Model file for the job. Use its own axes, mm. Face numbers are marked on the shaded views. A direction names the side the tool comes from. Round coordinates to 2 decimals unless told otherwise and drop trailing zeros. Order: outer loops, then holes, each group sorted by start corner. A loop starts at its lowest first (then second) coordinate and runs counter-clockwise, first axis right, second up. Notation, with made-up numbers: (-4.75, 20) - (54.25, 20) arc R29 cw to (54.25, 56) - close; hole circle Ø9 at (88, 75.5). An arc over 180 degrees is marked (long way). Answer as CSV lines item,"result". Start each with the question number.
1. Band-saw the part on B-B on z = -19.5. List the corners of the cut face in (x, y) (3 decimals).
2. Pull direction X, two halves, no side cores. Call the marked faces 6, 7 and 8: released by +X, released by -X, zero draft, split by the parting line, or undercut.
3. Wall check: line 1 along Z through (x, y) = (26, 30); line 2 along X through (y, z) = (65, -109); line 3 along Y through (x, z) = (8, -41). Give the ranges that are in metal, low to high. Write a range as [from, to].
4. Band-saw the part on A-A on y = 0. List the corners of the cut face in (x, z), then the cut area to 3 significant figures.
5. 3-axis set-ups, long thin cutter, end or side, ignore diameter. For the marked faces 1, 2, 3, 4 and 5: which of +Z, -Z, +X, -X, +Y, -Y reach the whole face in a straight line?
6. Band-saw the part on D-D on y = 53.5. List the corners of the cut face in (x, z).
7. Band-saw the part on C-C on x = 16. State how many separate pieces and enclosed holes the cut face has, then the cut area to 3 significant figures.
8. Pin check, flat tips, straight feed: pin 1 Ø13.5 at (x, y) = (14.5, 131) entering from +Z; pin 2 Ø22.5 at (x, z) = (-6.5, 131.5) entering from -Y; pin 3 Ø1.5 at (x, z) = (26, 98) entering from -Y. Stop position of each tip, or through.
```python
from build123d import *

# Parameters (mm, degrees)
BOSS_EXTRUDE1_DEPTH = 50
SKETCH4_R           = 150
SKETCH4_R_2         = 100
BOSS_EXTRUDE3_DEPTH = 100
CUT_EXTRUDE1_DEPTH  = 120
SKETCH7_R           = 150
SKETCH7_R_2         = 105
BOSS_EXTRUDE6_DEPTH = 4


with BuildPart() as part:
    # Sketch2 → Boss-Extrude1 (new, symmetric)
    with BuildSketch(Plane.YZ):
        with BuildLine():
            Line((-24.368621785, -28.502987077), (-80.352540378, -60.825317547))
            Line((-80.352540378, -60.825317547), (-92.852540378, -39.174682453))
            Line((-92.852540378, -39.174682453), (-36.868621785, -6.852351982))
            ThreePointArc((-36.868621785, -6.852351982), (-37.5, 0), (-36.868621785, 6.852351982))
            Line((-36.868621785, 6.852351982), (-92.852540378, 39.174682453))
            Line((-92.852540378, 39.174682453), (-80.352540378, 60.825317547))
            Line((-80.352540378, 60.825317547), (-24.368621785, 28.502987077))
            ThreePointArc((-24.368621785, 28.502987077), (-18.75, 32.475952642), (-12.5, 35.355339059))
            Line((-12.5, 35.355339059), (-12.5, 100))
            Line((-12.5, 100), (12.5, 100))
            Line((12.5, 100), (12.5, 35.355339059))
            ThreePointArc((12.5, 35.355339059), (18.75, 32.475952642), (24.368621785, 28.502987077))
            Line((24.368621785, 28.502987077), (80.352540378, 60.825317547))
            Line((80.352540378, 60.825317547), (92.852540378, 39.174682453))
            Line((92.852540378, 39.174682453), (36.868621785, 6.852351982))
            ThreePointArc((36.868621785, 6.852351982), (37.5, 0), (36.868621785, -6.852351982))
            Line((36.868621785, -6.852351982), (92.852540378, -39.174682453))
            Line((92.852540378, -39.174682453), (80.352540378, -60.825317547))
            Line((80.352540378, -60.825317547), (24.368621785, -28.502987077))
            ThreePointArc((24.368621785, -28.502987077), (18.75, -32.475952642), (12.5, -35.355339059))
            Line((12.5, -35.355339059), (12.5, -100))
            Line((12.5, -100), (-12.5, -100))
            Line((-12.5, -100), (-12.5, -35.355339059))
            ThreePointArc((-12.5, -35.355339059), (-18.75, -32.475952642), (-24.368621785, -28.502987077))
        make_face()
        Polygon((-14.43375673, -25), (14.43375673, -25), (28.867513459, 0), (14.43375673, 25), (-14.43375673, 25), (-28.867513459, 0), align=None, mode=Mode.SUBTRACT)
    extrude(amount=BOSS_EXTRUDE1_DEPTH, both=True)

    # Sketch4 → Boss-Extrude3 (add)
    with BuildSketch(Plane.YZ.offset(50)):
        with Locations(Location((0, 0, 0), (0, 0, 270))):
            Circle(SKETCH4_R)
        Circle(SKETCH4_R_2, mode=Mode.SUBTRACT)
    extrude(amount=-BOSS_EXTRUDE3_DEPTH)

    # Sketch5 → Cut-Extrude1 (cut)
    with BuildSketch(Plane.YZ.offset(50)):
        with BuildLine():
            ThreePointArc((-70.626450965, 77.697518777), (-40.181760398, 97.007350914), (-5, 104.880884817))
            Line((-5, 104.880884817), (-5, 149.916643506))
            ThreePointArc((-5, 149.916643506), (-57.402514855, 138.581929877), (-102.47154133, 109.542609142))
            Line((-102.47154133, 109.542609142), (-70.626450965, 77.697518777))
        make_face()
        with BuildLine():
            Line((70.626450965, 77.697518777), (102.47154133, 109.542609142))
            ThreePointArc((102.47154133, 109.542609142), (57.402514855, 138.581929877), (5, 149.916643506))
            Line((5, 149.916643506), (5, 104.880884817))
            ThreePointArc((5, 104.880884817), (40.181760398, 97.007350914), (70.626450965, 77.697518777))
        make_face()
        with BuildLine():
            ThreePointArc((149.916643506, 5), (138.581929877, 57.402514855), (109.542609142, 102.47154133))
            Line((109.542609142, 102.47154133), (77.697518777, 70.626450965))
            ThreePointArc((77.697518777, 70.626450965), (97.007350914, 40.181760398), (104.880884817, 5))
            Line((104.880884817, 5), (149.916643506, 5))
        make_face()
        with BuildLine():
            Line((149.916643506, -5), (104.880884817, -5))
            ThreePointArc((104.880884817, -5), (97.007350914, -40.181760398), (77.697518777, -70.626450965))
            Line((77.697518777, -70.626450965), (109.542609142, -102.47154133))
            ThreePointArc((109.542609142, -102.47154133), (138.581929877, -57.402514855), (149.916643506, -5))
        make_face()
        with BuildLine():
            Line((102.47154133, -109.542609142), (70.626450965, -77.697518777))
            ThreePointArc((70.626450965, -77.697518777), (40.181760398, -97.007350914), (5, -104.880884817))
            Line((5, -104.880884817), (5, -149.916643506))
            ThreePointArc((5, -149.916643506), (57.402514855, -138.581929877), (102.47154133, -109.542609142))
        make_face()
        with BuildLine():
            Line((-5, -149.916643506), (-5, -104.880884817))
            ThreePointArc((-5, -104.880884817), (-40.181760398, -97.007350914), (-70.626450965, -77.697518777))
            Line((-70.626450965, -77.697518777), (-102.47154133, -109.542609142))
            ThreePointArc((-102.47154133, -109.542609142), (-57.402514855, -138.581929877), (-5, -149.916643506))
        make_face()
        with BuildLine():
            ThreePointArc((-77.697518777, -70.626450965), (-97.007350914, -40.181760398), (-104.880884817, -5))
            Line((-104.880884817, -5), (-149.916643506, -5))
            ThreePointArc((-149.916643506, -5), (-138.581929877, -57.402514855), (-109.542609142, -102.47154133))
            Line((-109.542609142, -102.47154133), (-77.697518777, -70.626450965))
        make_face()
        with BuildLine():
            ThreePointArc((-104.880884817, 5), (-97.007350914, 40.181760398), (-77.697518777, 70.626450965))
            Line((-77.697518777, 70.626450965), (-109.542609142, 102.47154133))
            ThreePointArc((-109.542609142, 102.47154133), (-138.581929877, 57.402514855), (-149.916643506, 5))
            Line((-149.916643506, 5), (-104.880884817, 5))
        make_face()
    extrude(amount=-CUT_EXTRUDE1_DEPTH, mode=Mode.SUBTRACT)

    # Sketch7 → Boss-Extrude6 (add)
    with BuildSketch(Plane.YZ.offset(50)):
        with Locations(Location((0, 0, 0), (0, 0, 270))):
            Circle(SKETCH7_R)
        Circle(SKETCH7_R_2, mode=Mode.SUBTRACT)
    boss_extrude6 = extrude(amount=-BOSS_EXTRUDE6_DEPTH)

    # Mirror2: Boss-Extrude6 across plane
    add(boss_extrude6.mirror(Plane(origin=(0, 0, 0), x_dir=(0, 0, 1), z_dir=(1, 0, 0))))


solid = part.part
```
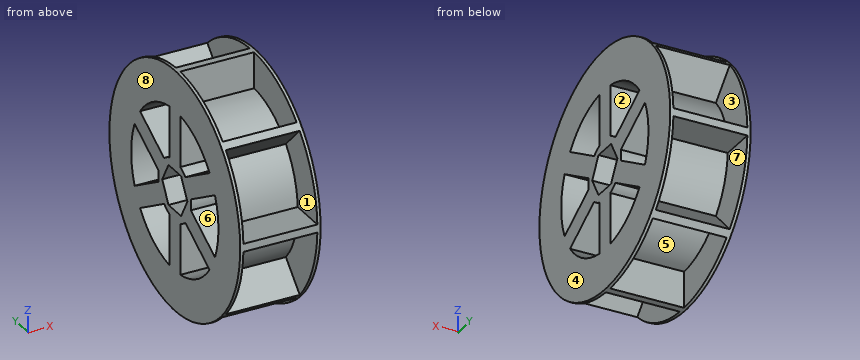
Reply:
1,outline,"(-50, -148.727) - (-46, -148.727) - (-46, -103.173) - (46, -103.173) - (46, -148.727) - (50, -148.727) - (50, -98.08) - (-50, -98.08) - close; (-50, -58.775) - (50, -58.775) - (50, -17.609) - (-50, -17.609) - close; (-50, 17.609) - (50, 17.609) - (50, 58.775) - (-50, 58.775) - close; (-50, 98.08) - (50, 98.08) - (50, 148.727) - (46, 148.727) - (46, 103.173) - (-46, 103.173) - (-46, 148.727) - (-50, 148.727) - close"
2,face 6,"zero draft"
2,face 7,"undercut"
2,face 8,"released by -X"
3,line 1,"z = [-100.62, -95.39], [-31.75, 31.75], [95.39, 100.62]"
3,line 2,"x = [-50, -46], [46, 50]"
3,line 3,"y = [-96.66, -46.01], [-12.5, 12.5], [46.01, 96.66]"
4,outline,"(-50, -150) - (50, -150) - (50, -25) - (-50, -25) - close; (-50, 25) - (50, 25) - (50, 150) - (-50, 150) - close"
4,area,"25,000 mm2"
5,face 1,"-Y"
5,face 2,"+X, -X"
5,face 3,"+Y"
5,face 4,"+Z, -Z, +X, +Y, -Y"
5,face 5,"-Z"
6,outline,"(-50, -140.13) - (-46, -140.13) - (-46, -90.35) - (46, -90.35) - (46, -140.13) - (50, -140.13) - (50, -84.49) - (-50, -84.49) - close; (-50, -45.32) - (50, -45.32) - (50, -16.45) - (-50, -16.45) - close; (-50, 16.45) - (50, 16.45) - (50, 45.32) - (-50, 45.32) - close; (-50, 84.49) - (50, 84.49) - (50, 140.13) - (46, 140.13) - (46, 90.35) - (-46, 90.35) - (-46, 140.13) - (-50, 140.13) - close"
7,separate pieces,"1"
7,enclosed holes,"7"
7,area,"18,500 mm2"
8,pin 1,"stops at z = 5"
8,pin 2,"stops at y = -5"
8,pin 3,"stops at y = -105.82"
